from build123d import *

# Parameters (mm, degrees)
SKETCH2_R           = 24.97201
SKETCH2_R_2         = 23.38451
EXTRUDE_THIN1_DEPTH = 1054.1
SKETCH4_R           = 3.175
CUT_EXTRUDE1_DEPTH  = 25.97201


with BuildPart() as part:
    # Sketch2 → Extrude-Thin1 (new body)
    with BuildSketch(Plane(origin=(0, 0, 0), x_dir=(1, 0, 0), z_dir=(0, 1, 0))):
        Circle(SKETCH2_R)
        Circle(SKETCH2_R_2, mode=Mode.SUBTRACT)
    extrude(amount=EXTRUDE_THIN1_DEPTH)

    # Sketch4 → Cut-Extrude1 (cut, symmetric)
    with BuildSketch(Plane(origin=(0, 0, 0), x_dir=(0, 0, -1), z_dir=(1, 0, 0))):
        with Locations((0, 1041.4)):
            Circle(SKETCH4_R)
    cut_extrude1 = extrude(amount=CUT_EXTRUDE1_DEPTH, both=True, mode=Mode.SUBTRACT)

    # Mirror1: Cut-Extrude1 across plane
    add(cut_extrude1.mirror(Plane.ZX.offset(527.05)), mode=Mode.SUBTRACT)


solid = part.part
Model file for the job. Use its own axes, mm. Give positions to 0.01 mm unless a question says otherwise; leave off trailing zeros. Order: outer loops, then holes, each group sorted by start corner. A loop starts at its lowest first (then second) coordinate and runs counter-clockwise, first axis right, second up. Notation, with made-up numbers: (68.25, 14.5) - (126.25, 14.5) arc R22 ccw to (126.25, 38.5) - close; hole circle Ø10 at (68, 44.5). An arc over 180 degrees is marked (long way). Write item = value, one per line. Start each with the question number.
1. Drop flat-ended pins along their axis: P1, Ø1, axis at x = 9.5, y = 917, coming from the -Z side; P2, Ø10, axis at x = 2.5, y = 353.5, coming from the -Z side; P3, Ø10, axis at y = 12.7, z = 0, coming from the -X side; P4, Ø2, axis at x = -3.5, y = 308, coming from the +Z side. Give the stop position or say it passes through.
2. Two-plate mould, pull along Z, no slides. Class faces 1 (the flat face through (-7.52, 0, -22.31)), 2 (the cylindrical face through (-3.25, 519.67, -24.76)), 3 (the cylindrical face through (22.305, 519.671, -7.024)): pulls with the +Z half, pulls with the -Z half, needs draft (parallel to the pull), parting line crosses it, or undercut.
3. Cut at B-B, the plane z = 12. List the corners of the cut face in (x, y).
4. Cut at A-A, the plane x = 0. List the corners of the cut face in (y, z), and give its area (3 significant figures).
5. Cut at C-C, the plane y = 801. List the corners of the cut face in (x, z), and give its area (3 significant figures).
6. Probe line 1 along Y through (x, z) = (24, 0) (3 decimals); line 2 along Z through (x, y) = (1, 979.5); line 3 along X through (y, z) = (516, -1.5). List the from-to ranges inside material, lowest first.
Taken from the geometry:
q1.P1 = -23.29
q1.P2 = -24.97
q1.P3 = -24.97
q1.P4 = 24.85
q2.face_1 = needs draft
q2.face_2 = parting line crosses it
q2.face_3 = undercut
q3.outline = (-21.9, 0) - (-20.07, 0) - (-20.07, 1054.1) - (-21.9, 1054.1) - close; (20.07, 0) - (21.9, 0) - (21.9, 1054.1) - (20.07, 1054.1) - close
q4.outline = (0, -24.97) - (1054.1, -24.97) - (1054.1, -23.38) - (0, -23.38) - close; (0, 23.38) - (1054.1, 23.38) - (1054.1, 24.97) - (0, 24.97) - close
q4.area = 3,350 mm²
q5.outline = circle Ø49.94 at (0, 0); hole circle Ø46.77 at (0, 0)
q5.area = 241 mm²
q6.line_1 = 0 to 9.525, 15.875 to 1038.225, 1044.575 to 1054.1
q6.line_2 = -24.95 to -23.36, 23.36 to 24.95
q6.line_3 = -24.93 to -23.34, 23.34 to 24.93
